from build123d import *

# Parameters (mm, degrees)
SKETCH_1_R          = 2
EXTRUDE_1_DEPTH     = 5
SKETCH_2_R          = 3
CUT_EXTRUDE_1_DEPTH = 1
FILLET_1_R          = 0.5


with BuildPart() as part:
    # 草图1 → 凸台-拉伸1 (new body)
    with BuildSketch(Plane.XY):
        Polygon((4.041451884, 0), (2.020725942, 3.5), (-2.020725942, 3.5), (-4.041451884, 0), (-2.020725942, -3.5), (2.020725942, -3.5), align=None)
        Circle(SKETCH_1_R, mode=Mode.SUBTRACT)
    extrude(amount=EXTRUDE_1_DEPTH)

    # 草图2 → 切除-拉伸1 (cut)
    with BuildSketch(Plane.XY.offset(5)):
        Polygon((4.041451884, 0), (2.020725942, 3.5), (-2.020725942, 3.5), (-4.041451884, 0), (-2.020725942, -3.5), (2.020725942, -3.5), align=None)
        Circle(SKETCH_2_R, mode=Mode.SUBTRACT)
    extrude(amount=-CUT_EXTRUDE_1_DEPTH, mode=Mode.SUBTRACT)

    # 圆角1
    fillet_1_edges = [part.edges().sort_by_distance(p)[0] for p in [
        (-3, 0, 4),
    ]]
    fillet(fillet_1_edges, radius=FILLET_1_R - 0.0001)  # a hair under: the kernel refuses the full size


solid = part.part
The listing builds one solid part. Answer for the finished solid, in the listing's coordinates (mm). A direction names the side the tool comes from. Coordinates: 2 decimals unless noted, no trailing zeros. Write each loop counter-clockwise with the first axis right and the second up, starting at its lowest first coordinate (ties: lowest second). Pieces come first, ordered by that corner, then holes. Notation, with made-up numbers: M 63.5,-11.75 L 88.5,-11.75 A30 ccw 88.5,17.25 Z; hole C 66,-8.5 d3. An arc over 180 degrees is marked long. Use one line per item in the form item = value.
Item 1: Given P1, Ø3, axis at y = -2, z = 2.5, coming from the -X side, flat-ended and moving along its own axis, determine where the tip first touches the part or whether it passes through.
Model answer:
P1 = -3.75
Item 2: Find the intervals of material crossed by probe 1 along Y at (x, z) = (0, 4.7); probe 2 along Y at (x, z) = (0, 1.9); probe 3 along Z at (x, y) = (-2.25, 2.75), in increasing order.
Model answer:
probe_1 = -3 to -2, 2 to 3
probe_2 = -3.5 to -2, 2 to 3.5
probe_3 = 0 to 4
Item 3: For faces 1 (the face through (2, 2, 0)), 2 (the face through (-3, 0.1, 4.8)), determine the directions among +Z, -Z, +X, -X, +Y, -Y from which every point of the face is accessible in a straight line to the end or side of a thin tool.
Model answer:
face_1 = -Z, +X, -X, +Y, -Y
face_2 = +Z
Item 4: Find section B-B, the plane z = 1. Give the vertices of the cut face in (x, y).
Model answer:
outline = M -4.04,0 L -2.02,-3.5 L 2.02,-3.5 L 4.04,0 L 2.02,3.5 L -2.02,3.5 Z; hole C 0,0 d4
Item 5: The mould has two halves that part along Y. Classify faces 3 (the face through (3, -1.8, 2)), 4 (the face through (0, -2, 2)), 5 (the face through (-3, 1.8, 2)): released by +Y, released by -Y, zero draft, split by the parting line, or undercut.
Model answer:
face_3 = released by -Y
face_4 = undercut
face_5 = released by +Y
